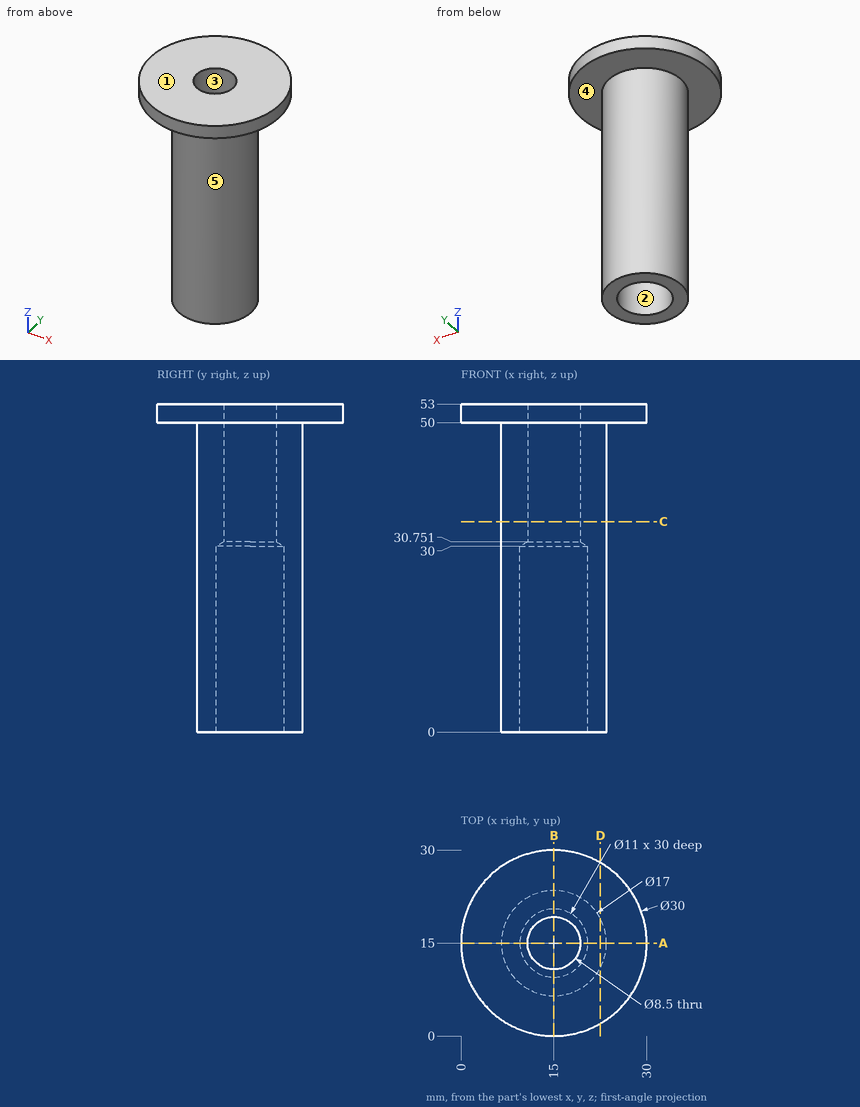
Here's the drawing with two shaded views (mm, measured from the low corner). I have some questions. A direction names the side the tool comes from. Give positions to 0.01 mm unless a question says otherwise; leave off trailing zeros. Write each loop counter-clockwise with the first axis right and the second up, starting at its lowest first coordinate (ties: lowest second). Pieces come first, ordered by that corner, then holes. Notation, with made-up numbers: (-25.75, -11.5) - (-3.75, -11.5) arc R20 ccw to (-3.75, 11.5) - close; hole circle Ø3 at (-29, 37.5). An arc over 180 degrees is marked (long way). Write item = value, one per line. Start each with the question number.
1. Imagine slicing it at C-C (z = 34). Please give me the cut outline in (x, y).
2. Thinking about a two-plate mould opening in X: for the marked faces 3, 4 and 5, which applies, released by +X, released by -X, zero draft, split by the parting line, or undercut?
3. Imagine slicing it at A-A (y = 15). Please give me the cut outline in (x, z), and give its area (3 significant figures).
4. Imagine slicing it at D-D (x = 22.5). Please give me the cut outline in (y, z), and give its area (3 significant figures).
5. On a 3-axis mill with a long thin cutter (end or side, diameter ignored), from which of +Z, -Z, +X, -X, +Y, -Y can I reach the whole of each face in a straight line? I mean the marked faces 1 and 2. Say none if no direction works.
6. Please list where these lines run through material, in increasing order: line 1 (Y direction, x = 15, z = 16); line 2 (Z direction, x = 26.25, y = 10.75); line 3 (Y direction, x = 18, z = 33).
7. For pin 1 (12 mm diameter, centred on x = 7.5, z = 43.5, fed in from +Y); pin 2 (3 mm diameter, centred on x = 15, y = 16.5, fed in from -Z); pin 3 (12 mm diameter, centred on y = 4, z = 11, fed in from +X); pin 4 (10 mm diameter, centred on y = 8.5, z = 14.5, fed in from +X), each with a flat end and sliding along its axis, tell me the tip position at first contact or that it passes through.
Worked answers:
q1.outline = circle Ø17 at (15, 15); hole circle Ø8.5 at (15, 15)
q2.face_3 = undercut
q2.face_4 = zero draft
q2.face_5 = split by the parting line
q3.outline = (0, 50) - (6.5, 50) - (6.5, 0) - (9.5, 0) - (9.5, 30) - (10.75, 30.75) - (10.75, 53) - (0, 53) - close; (19.25, 30.75) - (20.5, 30) - (20.5, 0) - (23.5, 0) - (23.5, 50) - (30, 50) - (30, 53) - (19.25, 53) - close
q3.area = 414 mm2
q4.outline = (2.01, 50) - (11, 50) - (11, 0) - (19, 0) - (19, 50) - (27.99, 50) - (27.99, 53) - (2.01, 53) - close
q4.area = 478 mm2
q5.face_1 = +Z, +X, -X, +Y, -Y
q5.face_2 = -Z
q6.line_1 = 6.5 to 9.5, 20.5 to 23.5
q6.line_2 = 50 to 53
q6.line_3 = 7.05 to 11.99, 18.01 to 22.95
q7.pin_1 = 23.37
q7.pin_2 = through
q7.pin_3 = 21.87
q7.pin_4 = 23.37
